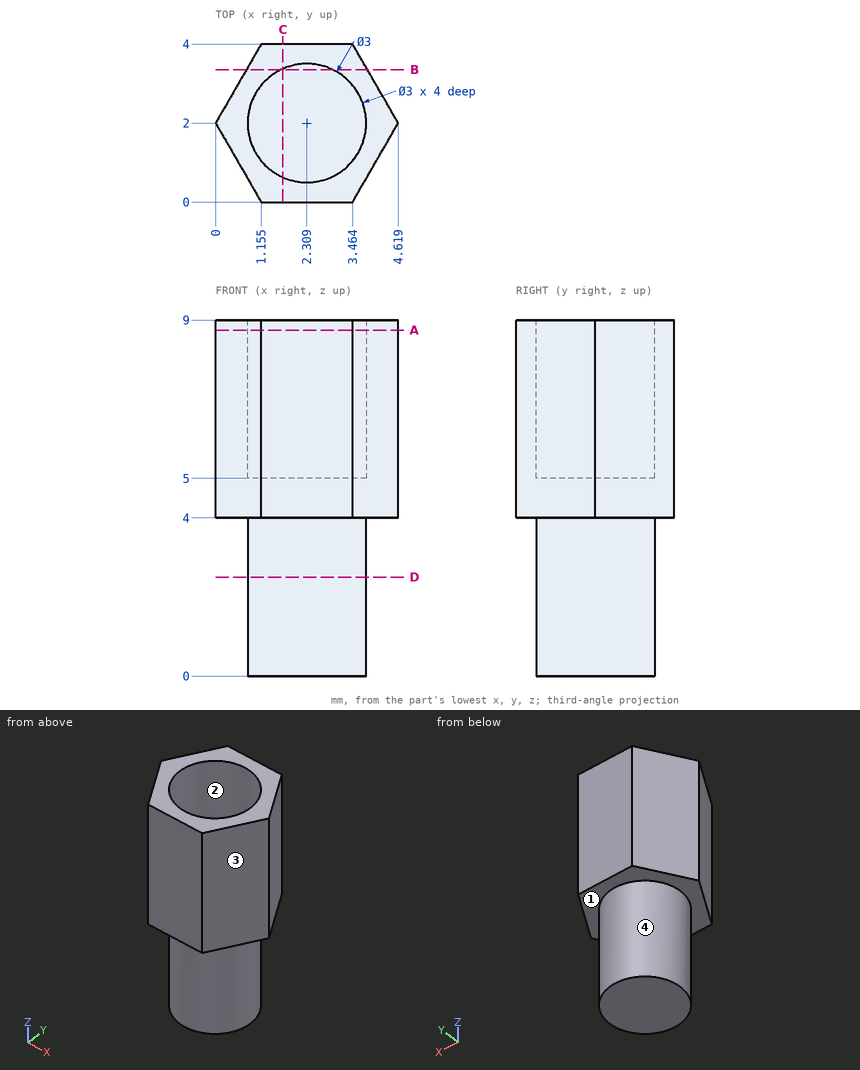
Print and shaded views of the part. All mm, measured from the part's lowest x, y and z. Give positions to 0.01 mm unless a question says otherwise; leave off trailing zeros. Write each loop counter-clockwise with the first axis right and the second up, starting at its lowest first coordinate (ties: lowest second). Pieces come first, ordered by that corner, then holes. Notation, with made-up numbers: (74, 41.5) - (126, 41.5) arc R12 cw to (126, 55.5) - close; hole circle Ø2 at (-21.5, -22.75). An arc over 180 degrees is marked (long way). One line per question, with ' | ' between items. Start each with the question number.
(1) Slice it at C-C on x = 1.7. Write the cut outline in (y, z), plus the area to 3 significant figures.
(2) Slice it at A-A on z = 8.75. Write the cut outline in (x, y) (1 decimal).
(3) Slice it at B-B on y = 3.35. Write the cut outline in (x, z) (1 decimal).
(4) Two-plate mould, pull along X, no slides. Class the marked faces 1, 2, 3 and 4: +X half, -X half, draft (parallel to the pull), parting line (faces both ways), or undercut.
(5) Wall check: line 1 along Z through (x, y) = (0.6, 2.7); line 2 along Y through (x, z) = (0.95, 7.5) (1 decimal); line 3 along Y through (x, z) = (2.4, 1). Give the ranges that are in metal, low to high. Write a range as from..to.
(6) Slice it at D-D on z = 2.5. Write the cut outline in (x, y).
Results below:
1) outline: (0, 4) - (0.63, 4) - (0.63, 0) - (3.37, 0) - (3.37, 4) - (4, 4) - (4, 9) - (3.37, 9) - (3.37, 5) - (0.63, 5) - (0.63, 9) - (0, 9) - close | area: 20.0 mm^2
2) outline: (0, 2) - (1.2, 0) - (3.5, 0) - (4.6, 2) - (3.5, 4) - (1.2, 4) - close; hole circle Ø3 at (2.3, 2)
3) outline: (0.8, 4) - (1.7, 4) - (1.7, 0) - (3, 0) - (3, 4) - (3.8, 4) - (3.8, 9) - (3, 9) - (3, 5) - (1.7, 5) - (1.7, 9) - (0.8, 9) - close
4) face 1: draft | face 2: undercut | face 3: +X half | face 4: parting line
5) line 1: 4..9 | line 2: 0.4..1.4, 2.6..3.6 | line 3: 0.5..3.5
6) outline: circle Ø3 at (2.31, 2)
